from build123d import *

# Parameters (mm, degrees)
SKETCH1_W           = 80.645
SKETCH1_H           = 112.395
SKETCH1_W_2         = 19.05
SKETCH1_H_2         = 38.1
BOSS_EXTRUDE1_DEPTH = 3.175
FILLET1_R           = 3.175


with BuildPart() as part:
    # Sketch1 → Boss-Extrude1 (new body)
    with BuildSketch(Plane.XY):
        Rectangle(SKETCH1_W, SKETCH1_H)
        with Locations((-8.5725, 0)):
            Rectangle(SKETCH1_W_2, SKETCH1_H_2, mode=Mode.SUBTRACT)
    extrude(amount=BOSS_EXTRUDE1_DEPTH)

    # Fillet1
    fillet1_edges = [part.edges().sort_by_distance(p)[0] for p in [
        (-18.0975, -19.05, 1.5875),
        (0.9525, -19.05, 1.5875),
        (0.9525, 19.05, 1.5875),
        (-18.0975, 19.05, 1.5875),
    ]]
    fillet(fillet1_edges, radius=FILLET1_R)


solid = part.part
Geometry: final body of the model. Coordinates: model frame, mm. A direction names the side the tool comes from. Coordinates: 2 decimals unless noted, no trailing zeros. Loops run counter-clockwise (first coordinate to the right, second up) from the corner with the lowest first, then second, coordinate; pieces in that order, holes last. Notation, with made-up numbers: (50.25, 42) - (104.25, 42) arc R27 ccw to (104.25, 70) - close; hole circle Ø7 at (52.5, -12). An arc over 180 degrees is marked (long way). Put each result on its own line as item: value. Start each with the question number.
Q1. Set-up query: faces 4 (the flat face through (8, 1, 3.175)), 5 (the cylindrical face through (0, -18.14, 1.61)). Return all of +Z, -Z, +X, -X, +Y, -Y with unobstructed straight access to the full face (end or side cutting, diameter ignored); none if empty.
Q2. Line query: line 1 (X direction, y = -11.5, z = 1.85). Output: solid intervals per line, ascending.
Q3. Cut plane B-B, the plane y = -1.5. Return loops of the section in (x, z) (1 decimal).
Q4. Pull-direction query (X, two-part tool) for faces 1 (the flat face through (40.322, -1, 2)), 2 (the flat face through (-18.098, 0, 2)), 3 (the flat face through (-40.322, -1, 2)); classes: released by +X, released by -X, zero draft, split by the parting line, or undercut.
Filled sheet:
1. face 4: +Z, +X, -X, +Y, -Y
1. face 5: +Z, -Z
2. line 1: -40.32 to -18.1, 0.95 to 40.32
3. outline: (-40.3, 0) - (-18.1, 0) - (-18.1, 3.2) - (-40.3, 3.2) - close; (1, 0) - (40.3, 0) - (40.3, 3.2) - (1, 3.2) - close
4. face 1: released by +X
4. face 2: undercut
4. face 3: released by -X
